```python
from build123d import *

# Parameters (mm, degrees)
F0_R     = 5
F1_DEPTH = 25


with BuildPart() as f1:
    # F0 (on Top) → F1 (new body)
    with BuildSketch(Plane.XY):
        with BuildLine():
            Line((39.869443, 53.510454), (30, 45))
            Line((30, 45), (-5, 45))
            ThreePointArc((-5, 45), (-28.584953, 31.928096), (-30, 5))
            Line((-30, 5), (-10.707767, -34.573811))
            ThreePointArc((-10.707767, -34.573811), (-4.008451, -42.087552), (5.627668, -45))
            Line((5.627668, -45), (30, -45))
            Line((30, -45), (41.184861, -53.695992))
            Line((41.184861, -53.695992), (55.873677, -53.695992))
            Line((55.873677, -53.695992), (55.873677, 53.510454))
            Line((55.873677, 53.510454), (39.869443, 53.510454))
        make_face()
        with Locations((30, -25.957934)):
            Circle(F0_R, mode=Mode.SUBTRACT)
        Circle(F0_R, mode=Mode.SUBTRACT)
        with Locations((30, 31.374168)):
            Circle(F0_R, mode=Mode.SUBTRACT)
    extrude(amount=F1_DEPTH)


solid = f1.part
```
Design review of the part built by this model. Coordinates are the model's own, in mm. A direction names the side the tool comes from. Round coordinates to 2 decimals unless told otherwise and drop trailing zeros. Write each loop counter-clockwise with the first axis right and the second up, starting at its lowest first coordinate (ties: lowest second). Pieces come first, ordered by that corner, then holes. Notation, with made-up numbers: (-6, -31.5) -> (18, -31.5) arc R14 ccw to (18, -17.5) -> close; hole circle Ø4 at (34, 40). An arc over 180 degrees is marked (long way). Answer in a Markdown table with one row per item.
Q1. Take a section at C-C, the plane z = 10.25. State the section outline as (x, y) points (1 decimal), then the cut area to 3 significant figures.
The answers:
| item | result |
|---|---|
| outline | (-30, 5) -> (-10.7, -34.6) arc R18.6 ccw to (5.6, -45) -> (30, -45) -> (41.2, -53.7) -> (55.9, -53.7) -> (55.9, 53.5) -> (39.9, 53.5) -> (30, 45) -> (-5, 45) arc R27.8 ccw to start; hole circle Ø10 at (0, 0); hole circle Ø10 at (30, -26); hole circle Ø10 at (30, 31.4) |
| area | 7,150 mm² |
Q2. To check wall thickness, follow L1, parallel to Y at x = 30, z = 6.25; L2, parallel to Y at x = 32, z = 19; L3, parallel to Y at x = 20, z = 18.5. State the ranges of each line that lie inside material, in increasing order. Write a range as [from, to].
The answers:
| item | result |
|---|---|
| L1 | [-45, -30.96], [-20.96, 26.37], [36.37, 45] |
| L2 | [-46.55, -30.54], [-21.38, 26.79], [35.96, 46.72] |
| L3 | [-45, 45] |
Q3. Take a section at B-B, the plane y = 0. State the section outline as (x, z) points, then the cut area to 3 significant figures.
The answers:
| item | result |
|---|---|
| outline | (-27.56, 0) -> (-5, 0) -> (-5, 25) -> (-27.56, 25) -> close; (5, 0) -> (55.87, 0) -> (55.87, 25) -> (5, 25) -> close |
| area | 1,840 mm² |
Q4. Take a section at A-A, the plane x = 28. State the section outline as (y, z) points, then the cut area to 3 significant figures.
The answers:
| item | result |
|---|---|
| outline | (-45, 0) -> (-30.54, 0) -> (-30.54, 25) -> (-45, 25) -> close; (-21.38, 0) -> (26.79, 0) -> (26.79, 25) -> (-21.38, 25) -> close; (35.96, 0) -> (45, 0) -> (45, 25) -> (35.96, 25) -> close |
| area | 1,790 mm² |
Q5. For faces 1 (the face through (13, 45, 12)), 2 (the face through (48, -53.696, 12)), 3 (the face through (18, -45, 12)), list the 3-axis set-ups (+Z, -Z, +X, -X, +Y, -Y) from which the entire face can be reached by the end or side of a thin tool; tool diameter is ignored.
The answers:
| item | result |
|---|---|
| face 1 | +Z, -Z, -X, +Y |
| face 2 | +Z, -Z, +X, -X, -Y |
| face 3 | +Z, -Z, -X, -Y |
Q6. Clearance check with flat-ended pins moving along their axes: pin 1 Ø12 at (x, z) = (21, 16) entering from -Y; pin 2 Ø1 at (x, z) = (-9.5, 2.5) entering from +Y; pin 3 Ø12 at (y, z) = (-28, 3) entering from -X; pin 4 Ø8 at (x, y) = (0, 0) entering from -Z. State where each tip first meets the part, or that it passes through.
The answers:
| item | result |
|---|---|
| pin 1 | y = -45 |
| pin 2 | y = 44.71 |
| pin 3 | x = -16.84 |
| pin 4 | through |
Q7. Draft analysis for pull direction X (two halves, no side actions). For faces 4 (the face through (48, 53.51, 12)), 5 (the face through (-1.08, -4.88, 12.32)), 6 (the face through (35.514, -49.287, 12.325)), state which applies: +X half, -X half, draft (parallel to the pull), parting line (faces both ways), or undercut.
The answers:
| item | result |
|---|---|
| face 4 | draft |
| face 5 | undercut |
| face 6 | -X half |
Q8. Take a section at D-D, the plane x = 38. State the section outline as (y, z) points.
The answers:
| item | result |
|---|---|
| outline | (-51.22, 0) -> (51.9, 0) -> (51.9, 25) -> (-51.22, 25) -> close |
